Design review of the part shown in the three views and the two pictorial views. Dimensions are in mm from the part's minimum x, y and z. A direction names the side the tool comes from. Give positions to 0.01 mm unless a question says otherwise; leave off trailing zeros. Order: outer loops, then holes, each group sorted by start corner. A loop starts at its lowest first (then second) coordinate and runs counter-clockwise, first axis right, second up. Notation, with made-up numbers: (69.25, 19.25) - (93.25, 19.25) arc R24 cw to (93.25, 41.25) - close; hole circle Ø6 at (9, 50). An arc over 180 degrees is marked (long way). Write each question's results on one line, items separated by ' | '. Start each with the question number.
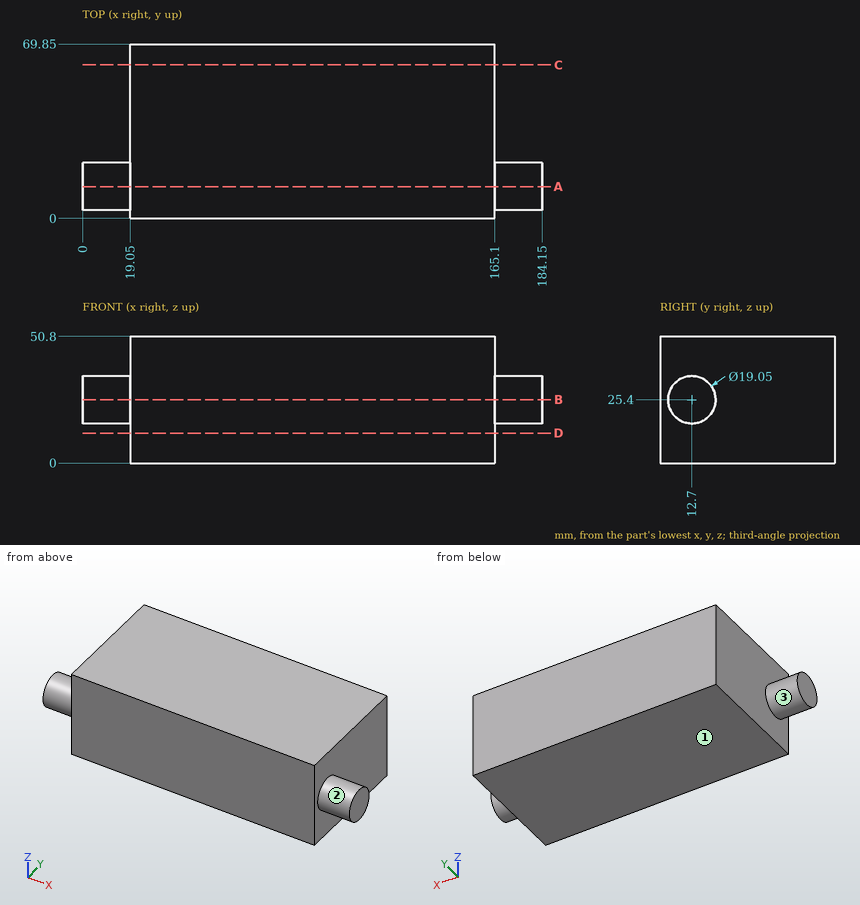
Q1. Machinability: for the marked faces 1, 2 and 3, which of the approach directions +Z, -Z, +X, -X, +Y, -Y give a long, thin tool a straight path to every point of the face, cutting with its end or side? Answer none if there is none.
Q2. Insertion check: pin 1 Ø1.5 at (x, z) = (143, 26) entering from -Y; pin 2 Ø4 at (y, z) = (52.5, 31.5) entering from +X. Each pin has a flat end and moves straight along its axis. Give the tip position at first contact, or say it passes through.
Q3. Add section A-A (y = 12.7). Give the boundary of the cut face in (x, z) (3 decimals).
Q4. For line 1 (X direction, y = 54, z = 46.5); line 2 (Z direction, x = 9, y = 15); line 3 (Y direction, x = 17, z = 28), list the stretches that pass through material, from the lowest coordinate up. Write a range as [from, to].
Q5. Add section B-B (z = 25.4). Give the boundary of the cut face in (x, y) (3 decimals), plus the area to 3 significant figures.
Q6. Add section C-C (y = 61.5). Give the boundary of the cut face in (x, z), plus the area to 3 significant figures.
Q7. Add section D-D (z = 12). Give the boundary of the cut face in (x, y).
Verdict:
1) face 1: -Z, +X, -X, +Y, -Y | face 2: +X | face 3: -X
2) pin 1: stops at y = 0 | pin 2: stops at x = 165.1
3) outline: (0, 15.875) - (19.05, 15.875) - (19.05, 0) - (165.1, 0) - (165.1, 15.875) - (184.15, 15.875) - (184.15, 34.925) - (165.1, 34.925) - (165.1, 50.8) - (19.05, 50.8) - (19.05, 34.925) - (0, 34.925) - close
4) line 1: x = [19.05, 165.1] | line 2: z = [16.16, 34.64] | line 3: y = [3.54, 21.86]
5) outline: (0, 3.175) - (19.05, 3.175) - (19.05, 0) - (165.1, 0) - (165.1, 3.175) - (184.15, 3.175) - (184.15, 22.225) - (165.1, 22.225) - (165.1, 69.85) - (19.05, 69.85) - (19.05, 22.225) - (0, 22.225) - close | area: 10,900 mm2
6) outline: (19.05, 0) - (165.1, 0) - (165.1, 50.8) - (19.05, 50.8) - close | area: 7,420 mm2
7) outline: (19.05, 0) - (165.1, 0) - (165.1, 69.85) - (19.05, 69.85) - close
